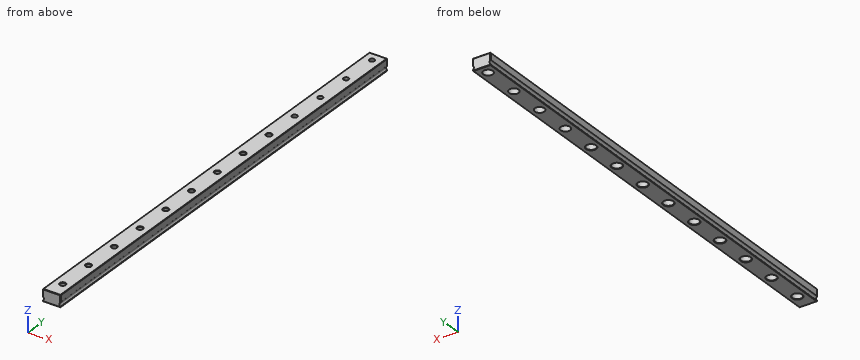
```python
from build123d import *

# Parameters (mm, degrees)
BOSS_EXTRUDE1_DEPTH = 317
SKETCH3_R           = 1.75
CUT_EXTRUDE3_DEPTH  = 8.5
SKETCH3_6_R         = 3.25
SKETCH3_6_R_2       = 1.75
CUT_EXTRUDE4_DEPTH  = 4.5
CHAMFER3_SIZE       = 0.25


with BuildPart() as part:
    # Sketch1 → Boss-Extrude1 (new body)
    with BuildSketch(Plane(origin=(0, 0, 0), x_dir=(1, 0, 0), z_dir=(0, 1, 0))):
        with BuildLine():
            Line((6, 4), (-6, 4))
            Line((-6, 4), (-6, 3.299038106))
            ThreePointArc((-6, 3.299038106), (-5.25, 2), (-6, 0.700961894))
            Line((-6, 0.700961894), (-6, -4))
            Line((-6, -4), (6, -4))
            Line((6, -4), (6, 0.700961894))
            ThreePointArc((6, 0.700961894), (5.25, 2), (6, 3.299038106))
            Line((6, 3.299038106), (6, 4))
        make_face()
    extrude(amount=BOSS_EXTRUDE1_DEPTH)

    # Sketch3 → Cut-Extrude3 (cut)
    with BuildSketch(Plane(origin=(0, 0, -4), x_dir=(-1, 0, 0), z_dir=(0, 0, -1))):
        with Locations((0, 335.75)):
            Circle(SKETCH3_R)
        with Locations((0, 310.75)):
            Circle(SKETCH3_R)
        with Locations((0, 285.75)):
            Circle(SKETCH3_R)
        with Locations((0, 260.75)):
            Circle(SKETCH3_R)
        with Locations((0, 235.75)):
            Circle(SKETCH3_R)
        with Locations((0, 210.75)):
            Circle(SKETCH3_R)
        with Locations((0, 185.75)):
            Circle(SKETCH3_R)
        with Locations((0, 160.75)):
            Circle(SKETCH3_R)
        with Locations((0, 110.75)):
            Circle(SKETCH3_R)
        with Locations((0, 85.75)):
            Circle(SKETCH3_R)
        with Locations((0, 60.75)):
            Circle(SKETCH3_R)
        with Locations((0, 35.75)):
            Circle(SKETCH3_R)
        with Locations((0, 135.75)):
            Circle(SKETCH3_R)
        with Locations((0, 10.75)):
            Circle(SKETCH3_R)
    extrude(amount=-CUT_EXTRUDE3_DEPTH, mode=Mode.SUBTRACT)

    # Sketch3<6> → Cut-Extrude4 (cut)
    # profile 1 of 14: a face of its own
    with BuildSketch(Plane(origin=(0, 0, -4), x_dir=(-1, 0, 0), z_dir=(0, 0, -1))):
        with Locations((0, 10.75)):
            Circle(SKETCH3_6_R)
        with Locations((0, 10.75)):
            Circle(SKETCH3_6_R_2, mode=Mode.SUBTRACT)
    # profile 2 of 14: a face of its own
    with BuildSketch(Plane(origin=(0, 0, -4), x_dir=(-1, 0, 0), z_dir=(0, 0, -1))):
        with Locations((0, 35.75)):
            Circle(SKETCH3_6_R)
        with Locations((0, 35.75)):
            Circle(SKETCH3_6_R_2, mode=Mode.SUBTRACT)
    # profile 3 of 14: a face of its own
    with BuildSketch(Plane(origin=(0, 0, -4), x_dir=(-1, 0, 0), z_dir=(0, 0, -1))):
        with Locations((0, 60.75)):
            Circle(SKETCH3_6_R)
        with Locations((0, 60.75)):
            Circle(SKETCH3_6_R_2, mode=Mode.SUBTRACT)
    # profile 4 of 14: a face of its own
    with BuildSketch(Plane(origin=(0, 0, -4), x_dir=(-1, 0, 0), z_dir=(0, 0, -1))):
        with Locations((0, 85.75)):
            Circle(SKETCH3_6_R)
        with Locations((0, 85.75)):
            Circle(SKETCH3_6_R_2, mode=Mode.SUBTRACT)
    # profile 5 of 14: a face of its own
    with BuildSketch(Plane(origin=(0, 0, -4), x_dir=(-1, 0, 0), z_dir=(0, 0, -1))):
        with Locations((0, 110.75)):
            Circle(SKETCH3_6_R)
        with Locations((0, 110.75)):
            Circle(SKETCH3_6_R_2, mode=Mode.SUBTRACT)
    # profile 6 of 14: a face of its own
    with BuildSketch(Plane(origin=(0, 0, -4), x_dir=(-1, 0, 0), z_dir=(0, 0, -1))):
        with Locations((0, 135.75)):
            Circle(SKETCH3_6_R)
        with Locations((0, 135.75)):
            Circle(SKETCH3_6_R_2, mode=Mode.SUBTRACT)
    # profile 7 of 14: a face of its own
    with BuildSketch(Plane(origin=(0, 0, -4), x_dir=(-1, 0, 0), z_dir=(0, 0, -1))):
        with Locations((0, 160.75)):
            Circle(SKETCH3_6_R)
        with Locations((0, 160.75)):
            Circle(SKETCH3_6_R_2, mode=Mode.SUBTRACT)
    # profile 8 of 14: a face of its own
    with BuildSketch(Plane(origin=(0, 0, -4), x_dir=(-1, 0, 0), z_dir=(0, 0, -1))):
        with Locations((0, 185.75)):
            Circle(SKETCH3_6_R)
        with Locations((0, 185.75)):
            Circle(SKETCH3_6_R_2, mode=Mode.SUBTRACT)
    # profile 9 of 14: a face of its own
    with BuildSketch(Plane(origin=(0, 0, -4), x_dir=(-1, 0, 0), z_dir=(0, 0, -1))):
        with Locations((0, 210.75)):
            Circle(SKETCH3_6_R)
        with Locations((0, 210.75)):
            Circle(SKETCH3_6_R_2, mode=Mode.SUBTRACT)
    # profile 10 of 14: a face of its own
    with BuildSketch(Plane(origin=(0, 0, -4), x_dir=(-1, 0, 0), z_dir=(0, 0, -1))):
        with Locations((0, 235.75)):
            Circle(SKETCH3_6_R)
        with Locations((0, 235.75)):
            Circle(SKETCH3_6_R_2, mode=Mode.SUBTRACT)
    # profile 11 of 14: a face of its own
    with BuildSketch(Plane(origin=(0, 0, -4), x_dir=(-1, 0, 0), z_dir=(0, 0, -1))):
        with Locations((0, 260.75)):
            Circle(SKETCH3_6_R)
        with Locations((0, 260.75)):
            Circle(SKETCH3_6_R_2, mode=Mode.SUBTRACT)
    # profile 12 of 14: a face of its own
    with BuildSketch(Plane(origin=(0, 0, -4), x_dir=(-1, 0, 0), z_dir=(0, 0, -1))):
        with Locations((0, 285.75)):
            Circle(SKETCH3_6_R)
        with Locations((0, 285.75)):
            Circle(SKETCH3_6_R_2, mode=Mode.SUBTRACT)
    # profile 13 of 14: a face of its own
    with BuildSketch(Plane(origin=(0, 0, -4), x_dir=(-1, 0, 0), z_dir=(0, 0, -1))):
        with Locations((0, 310.75)):
            Circle(SKETCH3_6_R)
        with Locations((0, 310.75)):
            Circle(SKETCH3_6_R_2, mode=Mode.SUBTRACT)
    # profile 14 of 14: a face of its own
    with BuildSketch(Plane(origin=(0, 0, -4), x_dir=(-1, 0, 0), z_dir=(0, 0, -1))):
        with Locations((0, 335.75)):
            Circle(SKETCH3_6_R)
        with Locations((0, 335.75)):
            Circle(SKETCH3_6_R_2, mode=Mode.SUBTRACT)
    extrude(amount=-CUT_EXTRUDE4_DEPTH, mode=Mode.SUBTRACT)

    # Chamfer3
    chamfer3_edges = [part.edges().sort_by_distance(p)[0] for p in [
        (-6, 0, 1.649519053),
        (1.75, 35.75, 0.5),
        (3.25, 35.75, -4),
        (-6, 0, -3.649519053),
        (1.75, 60.75, 0.5),
        (3.25, 60.75, -4),
        (1.75, 85.75, 0.5),
        (3.25, 85.75, -4),
        (0, 0, -4),
        (1.75, 110.75, 0.5),
        (3.25, 110.75, -4),
        (6, 0, -3.649519053),
        (1.75, 135.75, 0.5),
        (3.25, 135.75, -4),
        (1.75, 160.75, 0.5),
        (3.25, 160.75, -4),
        (1.75, 185.75, 0.5),
        (3.25, 185.75, -4),
        (1.75, 210.75, 0.5),
        (3.25, 210.75, -4),
        (0, 317, -4),
        (6, 158.5, 4),
        (-6, 158.5, 4),
        (-6, 158.5, -4),
        (6, 158.5, -4),
        (-6, 317, -3.649519053),
        (-6, 317, 1.649519053),
        (0, 317, 4),
        (6, 317, 1.649519053),
        (1.75, 210.75, 4),
        (1.75, 185.75, 4),
        (1.75, 60.75, 4),
        (1.75, 35.75, 4),
        (1.75, 135.75, 4),
        (1.75, 10.75, 4),
        (1.75, 85.75, 4),
        (1.75, 110.75, 4),
        (1.75, 160.75, 4),
        (6, 317, -3.649519053),
        (6, 0, 1.649519053),
        (1.75, 10.75, 0.5),
        (3.25, 10.75, -4),
        (0, 0, 4),
    ]]
    chamfer(chamfer3_edges, length=CHAMFER3_SIZE)


solid = part.part
```
For this review, take the finished solid that the model builds, in its own axes (mm). Coordinates: 2 decimals unless noted, no trailing zeros. Order: outer loops, then holes, each group sorted by start corner. A loop starts at its lowest first (then second) coordinate and runs counter-clockwise, first axis right, second up. Notation, with made-up numbers: (-9.75, 78.25) - (40.25, 78.25) arc R34 ccw to (40.25, 115.25) - close; hole circle Ø1 at (1.25, 83.5). An arc over 180 degrees is marked (long way). Answer as a JSON object with one key per item and string values. Group by question number.
1. We need section A-A on y = 145. State the section outline as (x, z) points.
2. For probe 1 along Z at (x, y) = (3, 186); probe 2 along X at (y, z) = (237, 2.5); probe 3 along X at (y, z) = (285, 0.25), list the stretches that pass through material, from the lowest coordinate up.
3. Clearance check with flat-ended pins moving along their axes: P1, Ø2, axis at x = 0, y = 35.75, coming from the +Z side; P2, Ø5, axis at x = 0, y = 235.75, coming from the -Z side. State where each tip first meets the part, or that it passes through.
Final values:
{
 "1": {"outline": "(-6, -3.75) - (-5.75, -4) - (5.75, -4) - (6, -3.75) - (6, -3.3) arc R1.5 cw to (6, -0.7) - (6, 3.75) - (5.75, 4) - (-5.75, 4) - (-6, 3.75) - (-6, -0.7) arc R1.5 cw to (-6, -3.3) - close"},
 "2": {"probe 1": "0.5 to 4", "probe 2": "-6 to -1.22, 1.22 to 6", "probe 3": "-6 to -3.16, 3.16 to 6"},
 "3": {"P1": "through", "P2": "z = 0.5"}
}
